The listing builds one solid part. Answer for the finished solid, in the listing's coordinates (mm). Coordinates: 2 decimals unless noted, no trailing zeros. Loops run counter-clockwise (first coordinate to the right, second up) from the corner with the lowest first, then second, coordinate; pieces in that order, holes last. Notation, with made-up numbers: M 86,48.25 L 144,48.25 A28 cw 144,87.25 Z; hole C 52.5,73.25 d6. An arc over 180 degrees is marked long. Answer as CSV lines item,"result". Start each with the question number.
```python
from build123d import *

# Parameters (mm, degrees)
PAD_DEPTH        = 1
POCKET_DEPTH     = 0.001
HOLE_D           = 1.75
HOLE_CSINK_D     = 3.3
HOLE_CSINK_ANGLE = 90
SKETCH005_R      = 4.9
HOLE003_DEPTH    = 1.001
SKETCH006_R      = 1.5
HOLE004_DEPTH    = 1.001


with BuildPart() as part:
    # Sketch → Pad (new body)
    with BuildSketch(Plane.XY):
        with BuildLine():
            Line((-51.8, 52.175), (51.8, 52.175))
            ThreePointArc((52.175, 51.8), (52.065165, 52.065165), (51.8, 52.175))
            Line((52.175, 51.8), (52.175, -51.8))
            ThreePointArc((51.8, -52.175), (52.065165, -52.065165), (52.175, -51.8))
            Line((51.8, -52.175), (-51.8, -52.175))
            ThreePointArc((-52.175, -51.8), (-52.065165, -52.065165), (-51.8, -52.175))
            Line((-52.175, -51.8), (-52.175, 51.8))
            ThreePointArc((-51.8, 52.175), (-52.065165, 52.065165), (-52.175, 51.8))
        make_face()
    extrude(amount=-PAD_DEPTH)

    # Sketch002 → Pocket (cut, through all)
    with BuildSketch(Plane.XY.offset(-4.8)):
        with BuildLine():
            Line((-45, 50.175), (45, 50.175))
            ThreePointArc((45, 50.175), (45.353553, 50.321447), (45.5, 50.675))
            ThreePointArc((45.5, 50.675), (45.353553, 51.028553), (45, 51.175))
            Line((-45, 51.175), (45, 51.175))
            ThreePointArc((-45, 51.175), (-45.353553, 51.028553), (-45.5, 50.675))
            ThreePointArc((-45.5, 50.675), (-45.353553, 50.321447), (-45, 50.175))
        make_face()
        with BuildLine():
            Line((-45, -51.175), (45, -51.175))
            ThreePointArc((45, -51.175), (45.353553, -51.028553), (45.5, -50.675))
            ThreePointArc((45.5, -50.675), (45.353553, -50.321447), (45, -50.175))
            Line((-45, -50.175), (45, -50.175))
            ThreePointArc((-45, -50.175), (-45.353553, -50.321447), (-45.5, -50.675))
            ThreePointArc((-45.5, -50.675), (-45.353553, -51.028553), (-45, -51.175))
        make_face()
        with BuildLine():
            Line((51.175, -45), (51.175, 45))
            ThreePointArc((51.175, 45), (51.028553, 45.353553), (50.675, 45.5))
            ThreePointArc((50.675, 45.5), (50.321447, 45.353553), (50.175, 45))
            Line((50.175, -45), (50.175, 45))
            ThreePointArc((50.175, -45), (50.321447, -45.353553), (50.675, -45.5))
            ThreePointArc((50.675, -45.5), (51.028553, -45.353553), (51.175, -45))
        make_face()
        with BuildLine():
            Line((-50.175, -45), (-50.175, 45))
            ThreePointArc((-50.175, 45), (-50.321447, 45.353553), (-50.675, 45.5))
            ThreePointArc((-50.675, 45.5), (-51.028553, 45.353553), (-51.175, 45))
            Line((-51.175, -45), (-51.175, 45))
            ThreePointArc((-51.175, -45), (-51.028553, -45.353553), (-50.675, -45.5))
            ThreePointArc((-50.675, -45.5), (-50.321447, -45.353553), (-50.175, -45))
        make_face()
    extrude(amount=-POCKET_DEPTH, mode=Mode.SUBTRACT)

    # Hole (through all)
    with Locations(Plane.XY):
        with Locations((-50, 50), (50, 50), (50, -50), (-50, -50)):
            CounterSinkHole(HOLE_D / 2, HOLE_CSINK_D / 2, counter_sink_angle=HOLE_CSINK_ANGLE)

    # Sketch005 → Hole003 (cut, through all)
    with BuildSketch(Plane.XY):
        with Locations((-40.005, 40.005)):
            Circle(SKETCH005_R)
        with Locations((-13.335, 40.005)):
            Circle(SKETCH005_R)
        with Locations((13.335, 40.005)):
            Circle(SKETCH005_R)
        with Locations((40.005, 40.005)):
            Circle(SKETCH005_R)
        with Locations((-40.005, 13.335)):
            Circle(SKETCH005_R)
        with Locations((-13.335, 13.335)):
            Circle(SKETCH005_R)
        with Locations((13.335, 13.335)):
            Circle(SKETCH005_R)
        with Locations((40.005, 13.335)):
            Circle(SKETCH005_R)
        with Locations((-40.005, -13.335)):
            Circle(SKETCH005_R)
        with Locations((-13.335, -13.335)):
            Circle(SKETCH005_R)
        with Locations((13.335, -13.335)):
            Circle(SKETCH005_R)
        with Locations((40.005, -13.335)):
            Circle(SKETCH005_R)
        with Locations((-40.005, -40.005)):
            Circle(SKETCH005_R)
        with Locations((-13.335, -40.005)):
            Circle(SKETCH005_R)
        with Locations((13.335, -40.005)):
            Circle(SKETCH005_R)
        with Locations((40.005, -40.005)):
            Circle(SKETCH005_R)
    extrude(amount=-HOLE003_DEPTH, mode=Mode.SUBTRACT)

    # Sketch006 → Hole004 (cut, through all)
    with BuildSketch(Plane.XY):
        with Locations((-40.005, 48.505)):
            Circle(SKETCH006_R)
        with Locations((-13.335, 48.505)):
            Circle(SKETCH006_R)
        with Locations((13.335, 48.505)):
            Circle(SKETCH006_R)
        with Locations((40.005, 48.505)):
            Circle(SKETCH006_R)
        with Locations((-40.005, 21.835)):
            Circle(SKETCH006_R)
        with Locations((-13.335, 21.835)):
            Circle(SKETCH006_R)
        with Locations((13.335, 21.835)):
            Circle(SKETCH006_R)
        with Locations((40.005, 21.835)):
            Circle(SKETCH006_R)
        with Locations((-40.005, -4.835)):
            Circle(SKETCH006_R)
        with Locations((-13.335, -4.835)):
            Circle(SKETCH006_R)
        with Locations((13.335, -4.835)):
            Circle(SKETCH006_R)
        with Locations((40.005, -4.835)):
            Circle(SKETCH006_R)
        with Locations((-40.005, -31.505)):
            Circle(SKETCH006_R)
        with Locations((-13.335, -31.505)):
            Circle(SKETCH006_R)
        with Locations((13.335, -31.505)):
            Circle(SKETCH006_R)
        with Locations((40.005, -31.505)):
            Circle(SKETCH006_R)
    extrude(amount=-HOLE004_DEPTH, mode=Mode.SUBTRACT)


solid = part.part
```
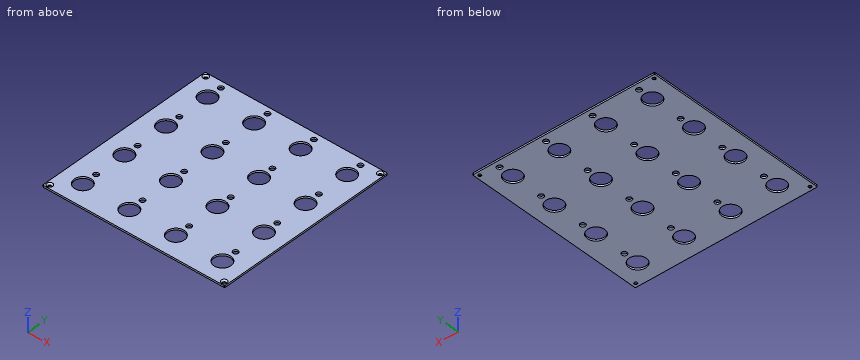
Item 1: Section A-A on y = 16.5 is taken. Determine the outline of the cut face in (x, z) (3 decimals), then the cut area to 3 significant figures.
Item 2: This flat-tipped pin is pushed along its axis until it touches: P1, Ø11.5, axis at x = 13.335, y = 40.005, coming from the -Z side. Where does it stop, or does it pass through?
Item 3: Section C-C on z = -0.5 is taken. State how many separate pieces and enclosed holes the cut face has, then the cut area to 3 significant figures.
Item 4: Section B-B on y = -11 is taken. Determine the outline of the cut face in (x, z) (3 decimals).
Item 5: Consider line 1 (Y direction, x = 50, z = -0.9) (3 decimals); line 2 (Y direction, x = -10.5, z = -0.45) (3 decimals); line 3 (X direction, y = -42, z = -0.6) (3 decimals). Determine where each line is inside the solid, lowest interval first.
Results are:
1,outline,"M -52.175,-1 L -43.746,-1 L -43.746,0 L -52.175,0 Z; M -36.264,-1 L -17.076,-1 L -17.076,0 L -36.264,0 Z; M -9.594,-1 L 9.594,-1 L 9.594,0 L -9.594,0 Z; M 17.076,-1 L 36.264,-1 L 36.264,0 L 17.076,0 Z; M 43.746,-1 L 52.175,-1 L 52.175,0 L 43.746,0 Z"
1,area,"74.4 mm²"
2,P1,"z = -1"
3,separate pieces,"1"
3,enclosed holes,"36"
3,area,"9,550 mm²"
4,outline,"M -52.175,-1 L -44.313,-1 L -44.313,0 L -52.175,0 Z; M -35.697,-1 L -17.643,-1 L -17.643,0 L -35.697,0 Z; M -9.027,-1 L 9.027,-1 L 9.027,0 L -9.027,0 Z; M 17.643,-1 L 35.697,-1 L 35.697,0 L 17.643,0 Z; M 44.313,-1 L 52.175,-1 L 52.175,0 L 44.313,0 Z"
5,line 1,"-52.175 to -50.875, -49.125 to 49.125, 50.875 to 52.175"
5,line 2,"-52.175 to -44.002, -36.008 to -17.332, -9.338 to 9.338, 17.332 to 36.008, 44.002 to 52.175"
5,line 3,"-52.175 to -44.48, -35.53 to -17.81, -8.86 to 8.86, 17.81 to 35.53, 44.48 to 52.175"
